```python
from build123d import *

# Parameters (mm, degrees)
F3_DEPTH = 17
F4_D     = 4.86


with BuildPart() as f1:
    # F0 (on Front) → F1 (revolve)
    with BuildSketch(Plane.XZ):
        Polygon((0, 30), (0, 0), (22.5, 0), (22.5, 25), (27.5, 25), (27.5, 30), align=None)
    revolve(axis=Axis((0, 0, 15), (0, 0, 1)))

    # F2 (on face) → F3 (cut)
    with BuildSketch(Plane.XY.offset(30)):
        with BuildLine():
            Line((2, -16.1), (0, -16.1))
            Line((0, -16.1), (-2, -16.1))
            Line((-2, -16.1), (-2, -18.190382))
            ThreePointArc((-2, -18.190382), (0, -18.3), (2, -18.190382))
            Line((2, -18.190382), (2, -16.1))
        make_face()
        with BuildLine():
            Line((0, -9.5), (0, 0))
            Line((0, 0), (0, 9.5))
            Line((0, 9.5), (0, 16.1))
            Line((0, 16.1), (-2, 16.1))
            Line((-2, 16.1), (-8.699425, 16.1))
            ThreePointArc((-8.699425, 16.1), (-18.3, 0), (-8.699425, -16.1))
            Line((-8.699425, -16.1), (-2, -16.1))
            Line((-2, -16.1), (0, -16.1))
            Line((0, -16.1), (0, -9.5))
        make_face()
        with BuildLine():
            Line((-2, 16.1), (0, 16.1))
            Line((0, 16.1), (2, 16.1))
            Line((2, 16.1), (2, 18.190382))
            ThreePointArc((2, 18.190382), (0, 18.3), (-2, 18.190382))
            Line((-2, 18.190382), (-2, 16.1))
        make_face()
        with BuildLine():
            Line((0, 9.5), (0, 0))
            Line((0, 0), (10, 0))
            Line((10, 0), (18.3, 0))
            ThreePointArc((18.3, 0), (15.717657, 9.37258), (8.699425, 16.1))
            Line((8.699425, 16.1), (2, 16.1))
            Line((2, 16.1), (0, 16.1))
            Line((0, 16.1), (0, 9.5))
        make_face()
        with BuildLine():
            Line((10, 0), (0, 0))
            Line((0, 0), (0, -9.5))
            Line((0, -9.5), (0, -16.1))
            Line((0, -16.1), (2, -16.1))
            Line((2, -16.1), (8.699425, -16.1))
            ThreePointArc((8.699425, -16.1), (15.717657, -9.37258), (18.3, 0))
            Line((18.3, 0), (10, 0))
        make_face()
    extrude(amount=-F3_DEPTH, mode=Mode.SUBTRACT)

    # F4 (through all)
    with Locations(Plane.XY.offset(30)):
        with Locations((0, 9.5), (0, -9.5)):
            Hole(F4_D / 2)


solid = f1.part
```
Verification items for the finished model (mm, model axes). A direction names the side the tool comes from. Round coordinates to 2 decimals unless told otherwise and drop trailing zeros. Order: outer loops, then holes, each group sorted by start corner. A loop starts at its lowest first (then second) coordinate and runs counter-clockwise, first axis right, second up. Notation, with made-up numbers: (6, -4.5) - (22, -4.5) arc R25 cw to (22, 25.5) - close; hole circle Ø10 at (60, -25.5). An arc over 180 degrees is marked (long way). Use CSV: the item, a comma, the result in double quotes.
(1) Gauge pin test, flat ends, axial feed: pin 1 Ø5.5 at (x, z) = (-5.5, 20) entering from +Y; pin 2 Ø5 at (y, z) = (-10, 24) entering from -X; pin 3 Ø6 at (y, z) = (19.5, 13.5) entering from -X; pin 4 Ø4.5 at (x, y) = (0, 9.5) entering from +Z. Record the tip position at first contact, or that the pin passes through.
Entries:
pin 1,"y = 22.33"
pin 2,"x = -26.4"
pin 3,"x = -15.3"
pin 4,"through"
(2) Section check B-B on x = 0. Record the boundary of the cut face in (y, z).
Entries:
outline,"(-27.5, 25) - (-22.5, 25) - (-22.5, 0) - (-11.93, 0) - (-11.93, 13) - (-18.3, 13) - (-18.3, 30) - (-27.5, 30) - close; (-7.07, 0) - (7.07, 0) - (7.07, 13) - (-7.07, 13) - close; (11.93, 0) - (22.5, 0) - (22.5, 25) - (27.5, 25) - (27.5, 30) - (18.3, 30) - (18.3, 13) - (11.93, 13) - close"
(3) Thickness scan on probe 1 along Y at (x, z) = (0, 2.5); probe 2 along Y at (x, z) = (1, 7.75); probe 3 along Y at (x, z) = (-9, 21.75). Record the ranges inside material, lowest first. Write a range as from..to.
Entries:
probe 1,"-22.5..-11.93, -7.07..7.07, 11.93..22.5"
probe 2,"-22.48..-11.71, -7.29..7.29, 11.71..22.48"
probe 3,"-20.62..-15.93, 15.93..20.62"
(4) Section check D-D on y = 20. Record the boundary of the cut face in (x, z).
Entries:
outline,"(-18.87, 25) - (-10.31, 25) - (-10.31, 0) - (10.31, 0) - (10.31, 25) - (18.87, 25) - (18.87, 30) - (-18.87, 30) - close"
(5) Section check C-C on y = 9.5. Record the boundary of the cut face in (x, z).
Entries:
outline,"(-25.81, 25) - (-20.4, 25) - (-20.4, 0) - (-2.43, 0) - (-2.43, 13) - (-15.64, 13) - (-15.64, 30) - (-25.81, 30) - close; (2.43, 0) - (20.4, 0) - (20.4, 25) - (25.81, 25) - (25.81, 30) - (15.64, 30) - (15.64, 13) - (2.43, 13) - close"
(6) Mould release check, pull along X, two halves, no side actions. Record for faces 3 (the face through (0, 18.3, 21.6)), 4 (the face through (10.382, -19.961, 12.675)), 5 (the face through (23, 0, 25)): released by +X, released by -X, zero draft, split by the parting line, or undercut.
Entries:
face 3,"undercut"
face 4,"split by the parting line"
face 5,"zero draft"
(7) Section check A-A on z = 23.5. Record the boundary of the cut face in (x, y).
Entries:
outline,"circle Ø45 at (0, 0); hole (-8.7, -16.1) - (-2, -16.1) - (-2, -18.19) arc R18.3 ccw to (2, -18.19) - (2, -16.1) - (8.7, -16.1) arc R18.3 ccw to (8.7, 16.1) - (2, 16.1) - (2, 18.19) arc R18.3 ccw to (-2, 18.19) - (-2, 16.1) - (-8.7, 16.1) arc R18.3 ccw to start"
(8) Access from +Z, -Z, +X, -X, +Y, -Y to the whole of each face (thin tool, end or side, straight path). Record for faces 1 (the face through (5, -16.1, 22)), 2 (the face through (6, -18, 30)).
Entries:
face 1,"+Z"
face 2,"+Z, +X, -X, +Y, -Y"
